Autodesk Inventor part; units mm, degrees
ref_plane "YZ Plane" through (0, 0, 0) normal (1, 0, 0) x (0, 1, 0)
ref_plane "XZ Plane" through (0, 0, 0) normal (0, 1, 0) x (-1, 0, 0)
ref_plane "XY Plane" through (0, 0, 0) normal (0, 0, 1) x (1, 0, 0)
ref_plane "작업 평면1" through (23.5, -8, -2) normal (1, 0, 0) x (0, 0, -1)
sketch "스케치1" plane through (23.5, -8, -2) normal (1, 0, 0) x (0, 0, -1)
  line L0 (0, 16) -> (-8.15, 16)
  line L1 (-8.15, 16) -> (-8.15, 10.6)
  line L2 (-8.15, 10.6) -> (-12.15, 10.6)
  line L3 (-13.15, 9.6) -> (-12.15, 10.6)
  line L4 (-13.15, 9.6) -> (-13.15, 6.4)
  line L5 (-12.15, 5.4) -> (-13.15, 6.4)
  line L6 (-12.15, 5.4) -> (-8.15, 5.4)
  line L7 (-8.15, 5.4) -> (-8.15, 0)
  line L8 (-8.15, 0) -> (0, 0)
  line L9 (0, 16) -> (8.35, 16)
  line L10 (8.35, 16) -> (8.35, 15)
  line L11 (8.35, 15) -> (7.35, 14)
  line L12 (6.35, 14) -> (6.35, 2)
  line L13 (6.35, 14) -> (7.35, 14)
  line L14 (0, 0) -> (8.35, 0)
  line L15 (8.35, 0) -> (8.35, 1)
  line L16 (8.35, 1) -> (7.35, 2)
  line L17 (6.35, 2) -> (7.35, 2)
  line L18 (0, 16) -> (-8.15, 16)
  line L19 (-8.15, 10.6) -> (-12.15, 10.6)
  line L20 (-8.15, 10.6) -> (-12.15, 10.6)
  line L21 (-12.15, 10.6) -> (-13.15, 9.6)
  line L22 (-13.15, 6.4) -> (-12.15, 5.4)
  point P0 (-2, 8)
  dimension "d1" = 8.35
sketch "스케치2" plane through (-23.5, 8, 6.15) normal (0, 0, 1) x (1, 0, 0)
  arc A0 (7.9209, -9.6) -> (7.9209, -6.4) centre (6, -8) ccw
  line L0 (39.0791, -9.6) -> (7.9209, -9.6)
  circle A1 centre (6, -8) radius 2.5
  circle A2 centre (41, -8) radius 2.5
  circle A3 centre (41, -8) radius 2.5
  point P0 (23.5, -8)
  point P1 (7.9209, -6.4)
extrude "돌출1" add sketch "스케치1" against normal up to surface (47 mm away)
extrude "돌출2" cut sketch "스케치2" along normal mid plane 50
sketch "스케치3" plane through (-15.5791, 1.6, 11.15) normal (0, 0, 1) x (1, 0, 0)
  line L0 (15.5791, -14.4593) -> (15.5791, 15.5737)
  line L1 (-7.9209, 4.4) -> (-7.9209, -7.6)
  line L2 (-7.9209, 4.4) -> (11.0791, 4.4)
  line L3 (11.0791, 4.4) -> (11.0791, -7.6)
  line L4 (11.0791, -7.6) -> (-7.9209, -7.6)
  line L5 (-7.9209, -7.6) -> (-7.9209, 4.4)
  line L6 (39.0791, 4.4) -> (39.0791, -7.6)
  line L7 (39.0791, 4.4) -> (20.0791, 4.4)
  line L8 (20.0791, 4.4) -> (20.0791, -7.6)
  line L9 (20.0791, -7.6) -> (39.0791, -7.6)
  line L10 (39.0791, -7.6) -> (39.0791, 4.4)
  point P0 (15.5791, -1.6)
  dimension "d9" = 19
extrude "돌출3" cut sketch "스케치3" against normal up to surface (5 mm away)
properties part number "Bearing Spacer_2mmUP"
The model under review builds one solid part; all positions refer to its coordinate system, in mm. A direction names the side the tool comes from. Round coordinates to 2 decimals unless told otherwise and drop trailing zeros. Loops run counter-clockwise (first coordinate to the right, second up) from the corner with the lowest first, then second, coordinate; pieces in that order, holes last.
Item 1: Take a section at D-D (x = 13). Write out the cut boundary in (y, z).
Determined:
outline: (-8, -10.35) - (-7, -10.35) - (-6, -9.35) - (-6, -8.35) - (6, -8.35) - (6, -9.35) - (7, -10.35) - (8, -10.35) - (8, 6.15) - (-8, 6.15) - close
Item 2: For line 1 (Y direction, x = -17.5, z = 1); line 2 (X direction, y = -1.5, z = -6.75); line 3 (Y direction, x = -20.5, z = -8.5), list the stretches that pass through material, from the lowest coordinate up.
Determined:
line 1: y = -8 to -2.5, 2.5 to 8
line 2: x = -23.5 to -19.5, -15.5 to 15.5, 19.5 to 23.5
line 3: y = -8 to -6, 6 to 8
Item 3: Mouldability with a two-part tool opening along X and no side actions: class faces 1 (the face through (-23.5, 0, -2)), 2 (the face through (-20, 0, -1)), 3 (the face through (0, 4, 6.15)) as released by +X, released by -X, zero draft, split by the parting line, or undercut.
Determined:
face 1: released by -X
face 2: undercut
face 3: zero draft
Item 4: For faces 4 (the face through (0, -2.6, 8)), 5 (the face through (0, 2.6, 8)), 6 (the face through (4.5, 0, 9)), 7 (the face through (0.33, -6.51, -9.86)), list the 3-axis set-ups (+Z, -Z, +X, -X, +Y, -Y) from which the entire face can be reached by the end or side of a thin tool; tool diameter is ignored.
Determined:
face 4: +Z, +X, -X, -Y
face 5: +Z, +X, -X, +Y
face 6: +Z, +X, +Y, -Y
face 7: -Z, +X, -X
Item 5: Clearance check with flat-ended pins moving along their axes: pin 1 Ø1.5 at (y, z) = (0, 9) entering from -X; pin 2 Ø9.5 at (x, y) = (-10.5, -1) entering from -Z; pin 3 Ø3 at (x, z) = (0, 8.5) entering from -Y. State where each tip first meets the part, or that it passes through.
Determined:
pin 1: stops at x = -4.5
pin 2: stops at z = -8.35
pin 3: stops at y = -2.6
Item 6: Take a section at B-B (x = -17.5). Write out the cut boundary in (y, z), then the cut area to 4 significant figures.
Determined:
outline: (-8, -10.35) - (-7, -10.35) - (-6, -9.35) - (-6, -8.35) - (-2.5, -8.35) - (-2.5, 6.15) - (-8, 6.15) - close; (2.5, -8.35) - (6, -8.35) - (6, -9.35) - (7, -10.35) - (8, -10.35) - (8, 6.15) - (2.5, 6.15) - close
area: 166.5 mm2
Item 7: Take a section at C-C (z = -4.25). Write out the cut boundary in (x, y).
Determined:
outline: (-23.5, -8) - (23.5, -8) - (23.5, 8) - (-23.5, 8) - close; hole circle Ø5 at (-17.5, 0); hole circle Ø5 at (17.5, 0)
Item 8: Take a section at A-A (y = 0). Write out the cut boundary in (x, z).
Determined:
outline: (-23.5, -8.35) - (-20, -8.35) - (-20, 6.15) - (-23.5, 6.15) - close; (-15, -8.35) - (15, -8.35) - (15, 6.15) - (4.5, 6.15) - (4.5, 11.15) - (-4.5, 11.15) - (-4.5, 6.15) - (-15, 6.15) - close; (20, -8.35) - (23.5, -8.35) - (23.5, 6.15) - (20, 6.15) - close
